The model under review builds one solid part; all positions refer to its coordinate system, in mm. Face numbers are marked on the shaded views. Give positions to 0.01 mm unless a question says otherwise; leave off trailing zeros. Loops run counter-clockwise (first coordinate to the right, second up) from the corner with the lowest first, then second, coordinate; pieces in that order, holes last. Notation, with made-up numbers: M 29,20 L 67,20 A20 cw 67,52 Z; hole C 29,48 d4. An arc over 180 degrees is marked long. Return JSON: item names as keys, results as strings. Group by question number.
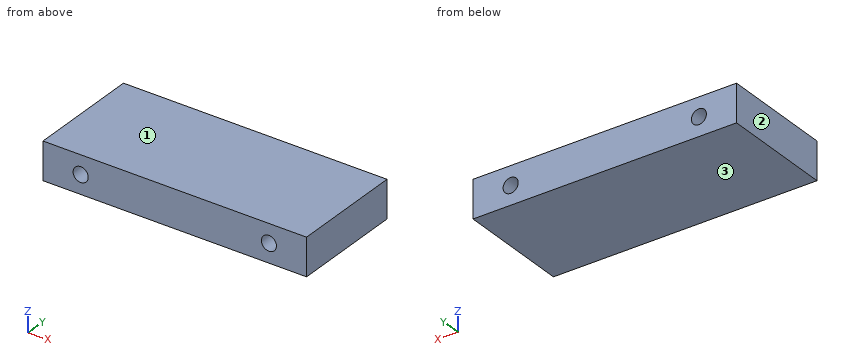
Autodesk Inventor part; units mm, degrees
ref_plane "YZ Plane" through (0, 0, 0) normal (1, 0, 0) x (0, 1, 0)
ref_plane "XZ Plane" through (0, 0, 0) normal (0, 1, 0) x (-1, 0, 0)
ref_plane "XY Plane" through (0, 0, 0) normal (0, 0, 1) x (1, 0, 0)
sketch "Sketch1" plane through (0, 0, 0) normal (0, 1, 0) x (-1, 0, 0)
  line L0 (33.2073, 5) -> (-36.7927, 5)
  line L1 (-36.7927, 5) -> (-36.7927, -5)
  line L2 (-36.7927, -5) -> (33.2073, -5)
  line L3 (33.2073, -5) -> (33.2073, 5)
  line L4 (33.2073, 5) -> (-36.7927, -5) construction
  line L5 (-36.7927, 5) -> (33.2073, -5) construction
  circle A0 centre (23.2073, 0) radius 2
  circle A1 centre (-26.7927, 0) radius 2
  point P0 (-1.7927, 0)
  point P1 (-1.7927, -5)
  dimension "d0" = 10
  dimension "d4" = 70
  dimension "d5" = 4
  dimension "d6" = 4
  dimension "d7" = 10
  dimension "d8" = 10
  dimension "d9" = 50
extrude "Extrusion1" add sketch "Sketch1" along normal blind 30
properties part number "Schiebegewicht Wand"
(1) Add section A-A (z = 0). Write out the cut boundary in (x, y).
(2) Mouldability with a two-part tool opening along Z and no side actions: class the marked faces 1, 2 and 3 as released by +Z, released by -Z, zero draft, split by the parting line, or undercut.
(3) Add section B-B (y = 15). Write out the cut boundary in (x, z).
(4) For pin 1 (3 mm diameter, centred on x = -23.21, z = 0, fed in from +Y), flat-tipped, find the tip position at first contact; note if it passes through.
(5) For probe 1 along Z at (x, y) = (27, 18.75); probe 2 along X at (y, z) = (5, 1); probe 3 along X at (y, z) = (6.25, -0.5), list the stretches that pass through material, from the lowest coordinate up.
Verdict:
{
 "1": {"outline": "M -33.21,0 L -25.21,0 L -25.21,30 L -33.21,30 Z; M -21.21,0 L 24.79,0 L 24.79,30 L -21.21,30 Z; M 28.79,0 L 36.79,0 L 36.79,30 L 28.79,30 Z"},
 "2": {"face 1": "released by +Z", "face 2": "zero draft", "face 3": "released by -Z"},
 "3": {"outline": "M -33.21,-5 L 36.79,-5 L 36.79,5 L -33.21,5 Z; hole C -23.21,0 d4; hole C 26.79,0 d4"},
 "4": {"pin 1": "passes through"},
 "5": {"probe 1": "z = -5 to -1.99, 1.99 to 5", "probe 2": "x = -33.21 to -24.94, -21.48 to 25.06, 28.52 to 36.79", "probe 3": "x = -33.21 to -25.14, -21.27 to 24.86, 28.73 to 36.79"}
}
